```python
from build123d import *

# Parameters (mm, degrees)
F1_DEPTH = 3
F2_W     = 20
F2_H     = 10
F3_DEPTH = 6
F4_W     = 20
F4_H     = 6
F5_DEPTH = 3
F6_W     = 20
F6_H     = 7
F7_DEPTH = 3


with BuildPart() as f1:
    # F0 (on Top) → F1 (new body)
    with BuildSketch(Plane.XY):
        with BuildLine():
            ThreePointArc((2.064754, -3.25858), (0, -2.122529), (-2.064754, -3.25858))
            Line((-2.064754, -3.25858), (-10, -15.781926))
            Line((-10, -15.781926), (-10, -42.324677))
            Line((-10, -42.324677), (0, -42.324677))
            Line((0, -42.324677), (10, -42.324677))
            Line((10, -42.324677), (10, -15.781926))
            Line((10, -15.781926), (2.064754, -3.25858))
        make_face()
        with BuildLine():
            ThreePointArc((-1.471273, -12.032518), (0, -10.824677), (1.471273, -12.032518))
            Line((1.471273, -12.032518), (3.080257, -20.135145))
            Line((3.080257, -20.135145), (-3.080257, -20.135145))
            Line((-3.080257, -20.135145), (-1.471273, -12.032518))
        make_face(mode=Mode.SUBTRACT)
    extrude(amount=F1_DEPTH)

    # F2 (on face) → F3 (join)
    with BuildSketch(Plane.XY.offset(3)):
        with Locations((0, -37.324677)):
            Rectangle(F2_W, F2_H)
    extrude(amount=F3_DEPTH)

    # F4 (on face) → F5 (cut)
    with BuildSketch(Plane(origin=(0, 0, 0), x_dir=(1, 0, 0), z_dir=(0, 0, -1))):
        with Locations((0, 39.324677)):
            Rectangle(F4_W, F4_H)
    extrude(amount=-F5_DEPTH, mode=Mode.SUBTRACT)

    # F6 (on face) → F7 (cut)
    with BuildSketch(Plane.XY.offset(9)):
        with Locations((0, -35.824677)):
            Rectangle(F6_W, F6_H)
    extrude(amount=-F7_DEPTH, mode=Mode.SUBTRACT)


solid = f1.part
```
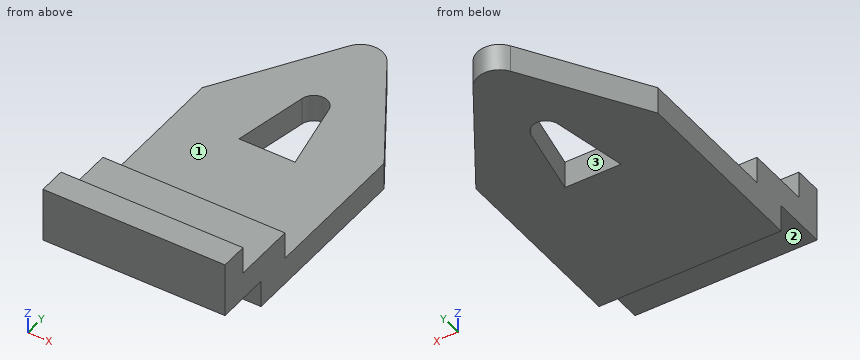
Check sheet for the modelled part. Datum: model origin and axes. Units: mm. Face numbers are marked on the shaded views. A direction names the side the tool comes from. Round coordinates to 2 decimals unless told otherwise and drop trailing zeros. Write each loop counter-clockwise with the first axis right and the second up, starting at its lowest first coordinate (ties: lowest second). Pieces come first, ordered by that corner, then holes. Notation, with made-up numbers: (-4.5, 3) -> (54.5, 3) arc R20 cw to (54.5, 11) -> close; hole circle Ø4 at (63.25, 31). An arc over 180 degrees is marked (long way). One line per question, with ' | ' between items. Start each with the question number.
1. Sectioned sample at B-B, the plane y = -11.5. Record the cut outline in (x, z), then the cut area to 3 significant figures.
2. Sectioned sample at A-A, the plane z = 1.25. Record the cut outline in (x, y), then the cut area to 3 significant figures.
3. Depth check by flat-ended pin: pin 1 (5 mm diameter, centred on x = 0, y = -40, fed in from -Z); pin 2 (3.5 mm diameter, centred on x = 1, y = -37.5, fed in from +Z); pin 3 (1.5 mm diameter, centred on x = -1, z = 2, fed in from +Y). Enter the tip coordinate at first touch or a pass-through.
4. Set-up check for the marked faces 1, 2 and 3: record each of +Z, -Z, +X, -X, +Y, -Y from which the full face is reachable in a straight line by a thin tool's end or side.
5. Sectioned sample at D-D, the plane z = 7. Record the cut outline in (x, y).
6. Scan lines: line 1 along Z through (x, y) = (6.5, -16); line 2 along Y through (x, z) = (9, 4.5); line 3 along Y through (x, z) = (-4, 8.75). Record each from-to range of solid material in increasing order. Write a range as from..to.
7. Sectioned sample at C-C, the plane x = -5.5. Record the cut outline in (y, z).
Taken from the geometry:
1) outline: (-7.29, 0) -> (-1.25, 0) -> (-1.25, 3) -> (-7.29, 3) -> close; (1.25, 0) -> (7.29, 0) -> (7.29, 3) -> (1.25, 3) -> close | area: 36.2 mm^2
2) outline: (-10, -36.32) -> (10, -36.32) -> (10, -15.78) -> (2.06, -3.26) arc R2.44 ccw to (-2.06, -3.26) -> (-10, -15.78) -> close; hole (-3.08, -20.14) -> (3.08, -20.14) -> (1.47, -12.03) arc R1.5 ccw to (-1.47, -12.03) -> close | area: 526 mm^2
3) pin 1: stops at z = 3 | pin 2: stops at z = 6 | pin 3: stops at y = -2.14
4) face 1: +Z, +X, -X, +Y | face 2: -Z, +X, -X, -Y | face 3: +Z, -Z
5) outline: (-10, -42.32) -> (10, -42.32) -> (10, -39.32) -> (-10, -39.32) -> close
6) line 1: z = 0..3 | line 2: y = -42.32..-32.32 | line 3: y = -42.32..-39.32
7) outline: (-42.32, 3) -> (-36.32, 3) -> (-36.32, 0) -> (-8.68, 0) -> (-8.68, 3) -> (-32.32, 3) -> (-32.32, 6) -> (-39.32, 6) -> (-39.32, 9) -> (-42.32, 9) -> close
